Verification items for the finished model (mm, model axes). A direction names the side the tool comes from. Round coordinates to 2 decimals unless told otherwise and drop trailing zeros. Write each loop counter-clockwise with the first axis right and the second up, starting at its lowest first coordinate (ties: lowest second). Pieces come first, ordered by that corner, then holes. Notation, with made-up numbers: (73.5, 77.5) - (82.5, 77.5) arc R9 ccw to (82.5, 93.5) - close; hole circle Ø11 at (-4.75, 19). An arc over 180 degrees is marked (long way). Answer as a JSON object with one key per item and string values.
```python
from build123d import *

# Parameters (mm, degrees)
SKETCH1_R                = 4.7
BOSS_EXTRUDE1_DEPTH      = 4
SKETCH2_R                = 3.95
BOSS_EXTRUDE2_DEPTH      = 6.5
SKETCH3_R                = 3.95
BOSS_EXTRUDE3_DEPTH      = 1
SKETCH4_R                = 3.95
BOSS_EXTRUDE4_DEPTH      = 2.5
SKETCH5_R                = 2.5
CUT_EXTRUDE1_DEPTH       = 16.497741771
CUT_EXTRUDE_1_DEPTH      = 0.2
CUT_EXTRUDE_1_DEPTH_BACK = 0.2
SKETCH_1_OUTSIDE_W       = 15.262
SKETCH_1_OUTSIDE_H       = 15.262
SKETCH_1_OUTSIDE_R       = 3.74


with BuildPart() as part:
    # Sketch1 → Boss-Extrude1 (new body)
    with BuildSketch(Plane(origin=(0, 0, 0), x_dir=(1, 0, 0), z_dir=(0, 1, 0))):
        with Locations(Location((0, 0, 0), (0, 0, 270))):
            Circle(SKETCH1_R)
    extrude(amount=BOSS_EXTRUDE1_DEPTH)

    # Sketch2 → Boss-Extrude2 (add)
    with BuildSketch(Plane(origin=(0, 4, 0), x_dir=(1, 0, 0), z_dir=(0, 1, 0))):
        with Locations(Location((0, 0, 0), (0, 0, 90))):
            Circle(SKETCH2_R)
    extrude(amount=BOSS_EXTRUDE2_DEPTH)

    # Sketch3 → Boss-Extrude3 (add)
    with BuildSketch(Plane(origin=(0, 10.5, 0), x_dir=(1, 0, 0), z_dir=(0, 1, 0))):
        with Locations(Location((0, 0, 0), (0, 0, 90))):
            Circle(SKETCH3_R)
    extrude(amount=BOSS_EXTRUDE3_DEPTH)

    # Sketch4 → Boss-Extrude4 (add)
    with BuildSketch(Plane(origin=(0, 11.5, 0), x_dir=(1, 0, 0), z_dir=(0, 1, 0))):
        with Locations(Location((0, 0, 0), (0, 0, 90))):
            Circle(SKETCH4_R)
    extrude(amount=BOSS_EXTRUDE4_DEPTH)

    # Sketch5 → Cut-Extrude1 (cut, through all)
    with BuildSketch(Plane(origin=(0, 14, 0), x_dir=(1, 0, 0), z_dir=(0, 1, 0))):
        with Locations(Location((0, 0, 0), (0, 0, 270))):
            Circle(SKETCH5_R)
    extrude(amount=-CUT_EXTRUDE1_DEPTH, mode=Mode.SUBTRACT)

    # 草图1 outside → 切除-拉伸1 (cut, two sides: drawn at the far end of the back side and taken through both)
    with BuildSketch(Plane(origin=(0, 10.75, 0), x_dir=(1, 0, 0), z_dir=(0, 1, 0)).offset(-CUT_EXTRUDE_1_DEPTH_BACK)):
        Rectangle(SKETCH_1_OUTSIDE_W, SKETCH_1_OUTSIDE_H)
        with Locations(Location((0, 0, 0), (0, 0, 270))):
            Circle(SKETCH_1_OUTSIDE_R, mode=Mode.SUBTRACT)
    extrude(amount=CUT_EXTRUDE_1_DEPTH + CUT_EXTRUDE_1_DEPTH_BACK, mode=Mode.SUBTRACT)


solid = part.part
```
Q1. Section check B-B, the plane x = 0. Record the cut outline in (y, z), then the cut area to 3 significant figures.
Geometry check:
{"outline": "(0, -4.7) - (4, -4.7) - (4, -3.95) - (10.55, -3.95) - (10.55, -3.74) - (10.95, -3.74) - (10.95, -3.95) - (14, -3.95) - (14, -2.5) - (0, -2.5) - close; (0, 2.5) - (14, 2.5) - (14, 3.95) - (10.95, 3.95) - (10.95, 3.74) - (10.55, 3.74) - (10.55, 3.95) - (4, 3.95) - (4, 4.7) - (0, 4.7) - close", "area": "46.4 mm2"}
Q2. Set-up check for faces 1 (the flat face through (-2, 0, 2)), 2 (the cylindrical face through (-2.67, 12.45, 2.91)): record each of +Z, -Z, +X, -X, +Y, -Y from which the full face is reachable in a straight line by a thin tool's end or side.
Geometry check:
{"face 1": "+Z, -Z, +X, -X, -Y", "face 2": "+Y"}
Q3. Section check D-D, the plane x = 2.75. Record the cut outline in (y, z).
Geometry check:
{"outline": "(0, -3.81) - (4, -3.81) - (4, -2.84) - (10.55, -2.84) - (10.55, -2.53) - (10.95, -2.53) - (10.95, -2.84) - (14, -2.84) - (14, 2.84) - (10.95, 2.84) - (10.95, 2.53) - (10.55, 2.53) - (10.55, 2.84) - (4, 2.84) - (4, 3.81) - (0, 3.81) - close"}
Q4. Material ranges on line 1 along X through (y, z) = (7.75, 0); line 2 along Z through (x, y) = (0.25, 6); line 3 along X through (y, z) = (7.5, 2.25), recorded low to high. Write a range as [from, to].
Geometry check:
{"line 1": "x = [-3.95, -2.5], [2.5, 3.95]", "line 2": "z = [-3.94, -2.49], [2.49, 3.94]", "line 3": "x = [-3.25, -1.09], [1.09, 3.25]"}
Q5. Section check A-A, the plane z = 0. Record the cut outline in (x, y).
Geometry check:
{"outline": "(-4.7, 0) - (-2.5, 0) - (-2.5, 14) - (-3.95, 14) - (-3.95, 10.95) - (-3.74, 10.95) - (-3.74, 10.55) - (-3.95, 10.55) - (-3.95, 4) - (-4.7, 4) - close; (2.5, 0) - (4.7, 0) - (4.7, 4) - (3.95, 4) - (3.95, 10.55) - (3.74, 10.55) - (3.74, 10.95) - (3.95, 10.95) - (3.95, 14) - (2.5, 14) - close"}
Q6. Section check C-C, the plane y = 2.5. Record the cut outline in (x, z), then the cut area to 3 significant figures.
Geometry check:
{"outline": "circle Ø9.4 at (0, 0); hole circle Ø5 at (0, 0)", "area": "49.8 mm2"}
Q7. Release check for a two-part mould opening along Y. For faces 3 (the flat face through (3, 14, 0)), 4 (the cylindrical face through (-3.65, 10.75, -0.81)), 5 (the cylindrical face through (1.412, 1.972, 4.483)) record: released by +Y, released by -Y, zero draft, split by the parting line, or undercut.
Geometry check:
{"face 3": "released by +Y", "face 4": "undercut", "face 5": "zero draft"}
Q8. Gauge pin test, flat ends, axial feed: P1, Ø1, axis at y = 3.5, z = 2.5, coming from the -X side; P2, Ø2.5, axis at x = 0.5, z = 0, coming from the -Y side; P3, Ø3, axis at y = 7, z = -2.5, coming from the +X side. Record the tip position at first contact, or that the pin passes through.
Geometry check:
{"P1": "stops at x = -4.25", "P2": "passes through", "P3": "stops at x = 3.82"}
